Work out the finished part from the listing and answer in its coordinate system (mm). Face numbers are marked on the shaded views. A direction names the side the tool comes from. Round coordinates to 2 decimals unless told otherwise and drop trailing zeros. Order: outer loops, then holes, each group sorted by start corner. A loop starts at its lowest first (then second) coordinate and runs counter-clockwise, first axis right, second up. Notation, with made-up numbers: (56, 53.25) -> (86, 53.25) arc R27 ccw to (86, 77.25) -> close; hole circle Ø6 at (-25, -12.5). An arc over 180 degrees is marked (long way). Use a Markdown table: item, result. Add a question column.
Item 1: A cutting plane is placed at A-A, the plane x = 0. Determine the outline of the cut face in (y, z), plus the area to 3 significant figures.
Item 2: A tool of negligible diameter and unlimited length cuts with its end or side. For the marked faces 4, 5 and 6, from which of +Z, -Z, +X, -X, +Y, -Y can it reach the whole face along a straight path? Write none if from no direction.
Item 3: A cutting plane is placed at B-B, the plane y = 14. Determine the outline of the cut face in (x, z).
Item 4: Find the intervals of material crossed by L1, parallel to X at y = 13, z = 27.5; L2, parallel to Y at x = 10.5, z = 96; L3, parallel to X at y = 6, z = 14, in increasing order. Write a range as [from, to].
Item 5: Flat-ended cylindrical pins translate along their axes: P1, Ø1, axis at y = 4.5, z = 83, coming from the -X side; P2, Ø5, axis at x = -12.5, z = 67.5, coming from the -Y side; P3, Ø2, axis at x = 18.5, z = 56, coming from the +Y side. Find the tip coordinate at first contact, or state that the pin passes through.
Item 6: For a pull along Y with two mould halves and no side action, classify the marked faces 1, 2 and 3 as +Y half, -Y half, draft (parallel to the pull), parting line (faces both ways), or undercut.
Item 7: A cutting plane is placed at C-C, the plane x = -20. Determine the outline of the cut face in (y, z), plus the area to 3 significant figures.
from build123d import *

# Parameters (mm, degrees)
F0_W     = 46.2
F0_H     = 46.2
F1_DEPTH = 116
F0_W_2   = 60
F0_H_2   = 60
F2_DEPTH = 4
F3_R     = 4
F4_R     = 2
F6_R     = 7.75
F7_DEPTH = 80


with BuildPart() as f1:
    # F0 (on Top) → F1 (new body)
    with BuildSketch(Plane.XY):
        Polygon((27.65, 17.65), (27.65, 27.65), (-27.65, 27.65), (-27.65, 17.65), (-28.15, 17.65), (-28.15, 7.65), (-27.65, 7.65), (-27.65, -7.65), (-28.15, -7.65), (-28.15, -17.65), (-27.65, -17.65), (-27.65, -27.65), (-17.65, -27.65), (-17.65, -28.15), (-7.65, -28.15), (-7.65, -27.65), (7.65, -27.65), (7.65, -28.15), (17.65, -28.15), (17.65, -27.65), (27.65, -27.65), (27.65, -17.65), (28.15, -17.65), (28.15, -7.65), (27.65, -7.65), (27.65, 7.65), (28.15, 7.65), (28.15, 17.65), align=None)
        Rectangle(F0_W, F0_H, mode=Mode.SUBTRACT)
    extrude(amount=F1_DEPTH)

    # F0 (on Top) → F2 (join)
    with BuildSketch(Plane.XY):
        Rectangle(F0_W_2, F0_H_2)
        Polygon((-27.65, 27.65), (27.65, 27.65), (27.65, 17.65), (28.15, 17.65), (28.15, 7.65), (27.65, 7.65), (27.65, -7.65), (28.15, -7.65), (28.15, -17.65), (27.65, -17.65), (27.65, -27.65), (17.65, -27.65), (17.65, -28.15), (7.65, -28.15), (7.65, -27.65), (-7.65, -27.65), (-7.65, -28.15), (-17.65, -28.15), (-17.65, -27.65), (-27.65, -27.65), (-27.65, -17.65), (-28.15, -17.65), (-28.15, -7.65), (-27.65, -7.65), (-27.65, 7.65), (-28.15, 7.65), (-28.15, 17.65), (-27.65, 17.65), align=None, mode=Mode.SUBTRACT)
        Polygon((27.65, 17.65), (27.65, 27.65), (-27.65, 27.65), (-27.65, 17.65), (-28.15, 17.65), (-28.15, 7.65), (-27.65, 7.65), (-27.65, -7.65), (-28.15, -7.65), (-28.15, -17.65), (-27.65, -17.65), (-27.65, -27.65), (-17.65, -27.65), (-17.65, -28.15), (-7.65, -28.15), (-7.65, -27.65), (7.65, -27.65), (7.65, -28.15), (17.65, -28.15), (17.65, -27.65), (27.65, -27.65), (27.65, -17.65), (28.15, -17.65), (28.15, -7.65), (27.65, -7.65), (27.65, 7.65), (28.15, 7.65), (28.15, 17.65), align=None)
        Rectangle(F0_W, F0_H, mode=Mode.SUBTRACT)
    extrude(amount=-F2_DEPTH)

    # F3
    f3_edges = [f1.edges().sort_by_distance(p)[0] for p in [
        (-27.65, 27.65, 58),
        (-27.65, -27.65, 58),
        (27.65, -27.65, 58),
        (27.65, 27.65, 58),
        (30, 30, -2),
        (30, -30, -2),
        (-30, 30, -2),
        (-30, -30, -2),
    ]]
    fillet(f3_edges, radius=F3_R)

    # F4
    f4_edges = [f1.edges().sort_by_distance(p)[0] for p in [
        (30, 0, -4),
    ]]
    fillet(f4_edges, radius=F4_R)

    # F6 (on offset) → F7 (cut)
    with BuildSketch(Plane.XZ.offset(27.65)):
        with Locations((0, 50)):
            Circle(F6_R)
    extrude(amount=-F7_DEPTH, mode=Mode.SUBTRACT)


solid = f1.part
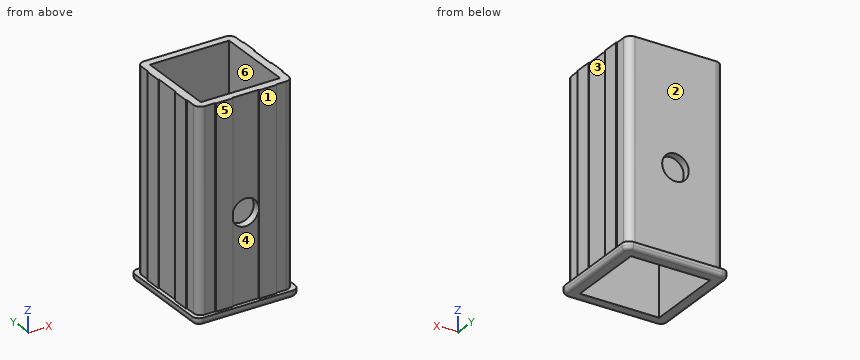
Reported:
| question | item | result |
|---|---|---|
| 1 | outline | (-30, -2) arc R2 ccw to (-28, -4) -> (-23.1, -4) -> (-23.1, 42.25) -> (-27.65, 42.25) -> (-27.65, 0) -> (-30, 0) -> close; (-27.65, 57.75) -> (-23.1, 57.75) -> (-23.1, 116) -> (-27.65, 116) -> close; (23.1, -4) -> (28, -4) arc R2 ccw to (30, -2) -> (30, 0) -> (27.65, 0) -> (27.65, 42.25) -> (23.1, 42.25) -> close; (23.1, 57.75) -> (27.65, 57.75) -> (27.65, 116) -> (23.1, 116) -> close |
| 1 | area | 968 mm² |
| 2 | face 4 | +Z, -Y |
| 2 | face 5 | +Z, +X, -X, -Y |
| 2 | face 6 | +Z, -Z |
| 3 | outline | (-30, -2) arc R2 ccw to (-28, -4) -> (-23.1, -4) -> (-23.1, 116) -> (-28.15, 116) -> (-28.15, 0) -> (-30, 0) -> close; (23.1, -4) -> (28, -4) arc R2 ccw to (30, -2) -> (30, 0) -> (28.15, 0) -> (28.15, 116) -> (23.1, 116) -> close |
| 4 | L1 | [-28.15, -23.1], [23.1, 28.15] |
| 4 | L2 | [-28.15, -23.1], [23.1, 27.65] |
| 4 | L3 | [-27.65, -23.1], [23.1, 27.65] |
| 5 | P1 | x = -27.65 |
| 5 | P2 | y = -28.15 |
| 5 | P3 | y = 27.65 |
| 6 | face 1 | -Y half |
| 6 | face 2 | +Y half |
| 6 | face 3 | undercut |
| 7 | outline | (-30, -2) arc R2 ccw to (-28, -4) -> (-23.1, -4) -> (-23.1, 116) -> (-27.65, 116) -> (-27.65, 0) -> (-30, 0) -> close; (23.1, -4) -> (28, -4) arc R2 ccw to (30, -2) -> (30, 0) -> (27.65, 0) -> (27.65, 116) -> (23.1, 116) -> close |
| 7 | area | 1,110 mm² |
